from build123d import *

# Parameters (mm, degrees)
F0_W     = 76.2
F0_H     = 50.8
F0_R     = 12.7
F1_DEPTH = 25.4
F2_W     = 10
F2_H     = 50.8
F3_DEPTH = 10
F2_W_2   = 12.7
F4_DEPTH = 8
F5_R     = 8.975174
F6_DEPTH = 30
F8_DEPTH = 50.8


with BuildPart() as f1:
    # F0 (on Top) → F1 (new body)
    with BuildSketch(Plane.XY):
        Rectangle(F0_W, F0_H)
        Circle(F0_R, mode=Mode.SUBTRACT)
    extrude(amount=-F1_DEPTH)

    # F2 (on Top) → F3 (cut)
    with BuildSketch(Plane.XY):
        with Locations((-30.56, 0)):
            Rectangle(F2_W, F2_H)
    extrude(amount=-F3_DEPTH, mode=Mode.SUBTRACT)

    # F2 (on Top) → F4 (cut)
    with BuildSketch(Plane.XY):
        Rectangle(F2_W_2, F2_H)
    extrude(amount=-F4_DEPTH, mode=Mode.SUBTRACT)

    # F5 (on face) → F6 (join)
    with BuildSketch(Plane.YZ.offset(38.1)):
        with Locations((0, -12.7)):
            Circle(F5_R)
    extrude(amount=F6_DEPTH)

    # F7 (on face) → F8 (cut)
    with BuildSketch(Plane.XZ.offset(25.4)):
        Polygon((31.75, 0), (19.05, 0), (16.117061, -5.08), (34.682939, -5.08), align=None)
    extrude(amount=-F8_DEPTH, mode=Mode.SUBTRACT)


solid = f1.part
The model under review builds one solid part; all positions refer to its coordinate system, in mm. A direction names the side the tool comes from. Give positions to 0.01 mm unless a question says otherwise; leave off trailing zeros. Write each loop counter-clockwise with the first axis right and the second up, starting at its lowest first coordinate (ties: lowest second). Pieces come first, ordered by that corner, then holes.
1. Add section D-D, the plane z = -1.75. Write out the cut boundary in (x, y).
2. Tool access review of faces 5 (the flat face through (6.35, -18, -4)), 6 (the flat face through (35, 0, 0)), 7 (the flat face through (25, 0, -5.08)): name each direction out of +Z, -Z, +X, -X, +Y, -Y from which nothing blocks a thin tool from reaching the whole face with its end or side.
3. Wall thickness on L1, parallel to X at y = 0, z = -6.5; L2, parallel to X at y = 0, z = -10.5; L3, parallel to X at y = -6, z = -4.25: over which ranges is each line inside the solid? List them lowest first.
4. Add section C-C, the plane z = -12.7. Write out the cut boundary in (x, y).
5. Add section B-B, the plane y = 0. Write out the cut boundary in (x, z).
6. Add section A-A, the plane x = 0. Write out the cut boundary in (y, z), plus the area to 3 significant figures.
7. Draft analysis for pull direction X (two halves, no side actions). For faces 1 (the flat face through (-6.35, 18, -4)), 2 (the flat face through (38.1, 5, -21)), 3 (the flat face through (0, 18, -8)), 4 (the flat face through (14, 0, 0)), state which applies: +X half, -X half, draft (parallel to the pull), parting line (faces both ways), or undercut.
8. For P1, Ø4, axis at y = 16, z = -3, coming from the +X side; P2, Ø9.5, axis at x = 22, y = -5.5, coming from the +Z side; P3, Ø3, axis at x = 48.5, y = 0.5, coming from the -Z side; P4, Ø6.5, axis at x = -3, y = -17.5, coming from the +Z side, all flat-tipped, find the tip position at first contact; note any pin that passes through.
Worked answers:
1. outline: (-38.1, -25.4) - (-35.56, -25.4) - (-35.56, 25.4) - (-38.1, 25.4) - close; (-25.56, -25.4) - (-6.35, -25.4) - (-6.35, -11) arc R12.7 cw to (-6.35, 11) - (-6.35, 25.4) - (-25.56, 25.4) - close; (6.35, -25.4) - (18.04, -25.4) - (18.04, 25.4) - (6.35, 25.4) - (6.35, 11) arc R12.7 cw to (6.35, -11) - close; (32.76, -25.4) - (38.1, -25.4) - (38.1, 25.4) - (32.76, 25.4) - close
2. face 5: +Z, +Y, -Y
2. face 6: +Z, +X, -X, +Y, -Y
2. face 7: +Y, -Y
3. L1: x = -38.1 to -35.56, -25.56 to -12.7, 12.7 to 68.1
3. L2: x = -38.1 to -12.7, 12.7 to 68.1
3. L3: x = -38.1 to -35.56, -25.56 to -11.19, 11.19 to 16.6, 34.2 to 38.1
4. outline: (-38.1, -25.4) - (38.1, -25.4) - (38.1, -8.98) - (68.1, -8.98) - (68.1, 8.98) - (38.1, 8.98) - (38.1, 25.4) - (-38.1, 25.4) - close; hole circle Ø25.4 at (0, 0)
5. outline: (-38.1, -25.4) - (-12.7, -25.4) - (-12.7, 0) - (-25.56, 0) - (-25.56, -10) - (-35.56, -10) - (-35.56, 0) - (-38.1, 0) - close; (12.7, -25.4) - (38.1, -25.4) - (38.1, -21.68) - (68.1, -21.68) - (68.1, -3.72) - (38.1, -3.72) - (38.1, 0) - (31.75, 0) - (34.68, -5.08) - (16.12, -5.08) - (19.05, 0) - (12.7, 0) - close
6. outline: (-25.4, -25.4) - (-12.7, -25.4) - (-12.7, -8) - (-25.4, -8) - close; (12.7, -25.4) - (25.4, -25.4) - (25.4, -8) - (12.7, -8) - close
6. area: 442 mm2
7. face 1: undercut
7. face 2: +X half
7. face 3: undercut
7. face 4: draft
8. P1: stops at x = 38.1
8. P2: stops at z = 0
8. P3: stops at z = -21.68
8. P4: stops at z = -8
